Work out the finished part from the listing and answer in its coordinate system (mm). A direction names the side the tool comes from. Coordinates: 2 decimals unless noted, no trailing zeros. Loops run counter-clockwise (first coordinate to the right, second up) from the corner with the lowest first, then second, coordinate; pieces in that order, holes last. Notation, with made-up numbers: (10.5, -25) -> (63.5, -25) arc R25 cw to (63.5, -5) -> close; hole circle Ø5 at (51, -2). An arc over 180 degrees is marked (long way). Use a Markdown table: item, result. Add a question column.
```python
from build123d import *

# Parameters (mm, degrees)
SKETCH026_R     = 30
PAD018_DEPTH    = 1.6
SKETCH027_R     = 7.9
SKETCH027_R_2   = 6.7
PAD019_DEPTH    = 6.4
SKETCH028_R     = 7.875
SKETCH028_R_2   = 6.7
PAD020_DEPTH    = 7.2
SKETCH029_R     = 6.7000000001
POCKET006_DEPTH = 1.601
CHAMFER008_SIZE = 0.6


with BuildPart() as part:
    # Sketch026 → Pad018 (new body)
    with BuildSketch(Plane.XY):
        Circle(SKETCH026_R)
    extrude(amount=PAD018_DEPTH)

    # Sketch027 → Pad019 (join)
    with BuildSketch(Plane.XY.offset(1.6)):
        Circle(SKETCH027_R)
        Circle(SKETCH027_R_2, mode=Mode.SUBTRACT)
    extrude(amount=PAD019_DEPTH)

    # Sketch028 → Pad020 (join)
    with BuildSketch(Plane.XY.offset(8)):
        Circle(SKETCH028_R)
        Circle(SKETCH028_R_2, mode=Mode.SUBTRACT)
    extrude(amount=PAD020_DEPTH)

    # Sketch029 → Pocket006 (cut, through all)
    with BuildSketch(Plane.XY.offset(1.6)):
        Circle(SKETCH029_R)
    extrude(amount=-POCKET006_DEPTH, mode=Mode.SUBTRACT)

    # Chamfer008
    chamfer008_edges = [part.edges().sort_by_distance(p)[0] for p in [
        (-7.9, 0, 1.6),
    ]]
    chamfer(chamfer008_edges, length=CHAMFER008_SIZE)


solid = part.part
```
Item 1: For a pull along X with two mould halves and no side action, classify faces 1 (the face through (-1.025, 7.808, 11.55)), 2 (the face through (6.2, -6.2, 1.6)) as +X half, -X half, draft (parallel to the pull), parting line (faces both ways), or undercut.
Item 2: Section A-A (y = 0) is taken. Determine the outline of the cut face in (x, z) (3 decimals), then the cut area to 3 significant figures.
Item 3: Find the intervals of material crossed by probe 1 along Y at (x, z) = (0, 0.9); probe 2 along Z at (x, y) = (14.5, 16.5); probe 3 along Y at (x, z) = (-3.5, 2.5), in increasing order.
Item 4: Section C-C (z = 11.25) is taken. Determine the outline of the cut face in (x, y) (3 decimals).
Item 5: Section D-D (y = -18) is taken. Determine the outline of the cut face in (x, z).
Item 6: Given pin 1 (1 mm diameter, centred on x = 9, z = 5.5, fed in from +Y); pin 2 (5 mm diameter, centred on x = -12, z = 2, fed in from -Y); pin 3 (5 mm diameter, centred on x = 7, z = 12, fed in from +Y); pin 4 (1 mm diameter, centred on y = 2, z = 5, fed in from -X), each flat-ended and moving along its own axis, determine where each tip first touches the part or whether it passes through.
Item 7: For faces 3 (the face through (-6.269, -4.807, 5.059)), 4 (the face through (2.3, 6.5, 15.2)), determine the directions among +Z, -Z, +X, -X, +Y, -Y from which every point of the face is accessible in a straight line to the end or side of a thin tool.
Output:
| question | item | result |
|---|---|---|
| 1 | face 1 | parting line |
| 1 | face 2 | draft |
| 2 | outline | (-30, 0) -> (-6.7, 0) -> (-6.7, 15.2) -> (-7.875, 15.2) -> (-7.875, 8) -> (-7.9, 8) -> (-7.9, 2.2) -> (-8.5, 1.6) -> (-30, 1.6) -> close; (6.7, 0) -> (30, 0) -> (30, 1.6) -> (8.5, 1.6) -> (7.9, 2.2) -> (7.9, 8) -> (7.875, 8) -> (7.875, 15.2) -> (6.7, 15.2) -> close |
| 2 | area | 107 mm2 |
| 3 | probe 1 | y = -30 to -6.7, 6.7 to 30 |
| 3 | probe 2 | z = 0 to 1.6 |
| 3 | probe 3 | y = -7.08 to -5.71, 5.71 to 7.08 |
| 4 | outline | circle Ø15.75 at (0, 0); hole circle Ø13.4 at (0, 0) |
| 5 | outline | (-24, 0) -> (24, 0) -> (24, 1.6) -> (-24, 1.6) -> close |
| 6 | pin 1 | passes through |
| 6 | pin 2 | stops at y = -28.45 |
| 6 | pin 3 | stops at y = 6.46 |
| 6 | pin 4 | stops at x = -7.76 |
| 7 | face 3 | +Z |
| 7 | face 4 | +Z, +X, -X, +Y, -Y |
